Read the model definition and answer for the solid it produces. Units are mm, in the model's axes. Face numbers are marked on the shaded views. A direction names the side the tool comes from. Give positions to 0.01 mm unless a question says otherwise; leave off trailing zeros. Loops run counter-clockwise (first coordinate to the right, second up) from the corner with the lowest first, then second, coordinate; pieces in that order, holes last. Notation, with made-up numbers: (-10.5, -36.5) - (26.5, -36.5) arc R22 ccw to (26.5, 2.5) - close; hole circle Ø4 at (-7, 88.5). An arc over 180 degrees is marked (long way). Write each question's results on one line, items separated by ' | '. Start each with the question number.
Q1. The part is cut by section D-D, the plane z = -15. State how many separate pieces and enclosed holes the cut face has, plus the area to 3 significant figures.
Q2. The part is cut by section A-A, the plane y = 15.06. Write down the section's boundary in (x, z) (3 decimals).
Q3. The part is cut by section B-B, the plane x = 16.5. Write down the section's boundary in (y, z), plus the area to 3 significant figures.
Q4. For the marked faces 4, 5, 6, 7 and 8, determine the directions among +Z, -Z, +X, -X, +Y, -Y from which every point of the face is accessible in a straight line to the end or side of a thin tool.
Q5. Given pin 1 (1.5 mm diameter, centred on x = 31, z = -11.5, fed in from -Y); pin 2 (15 mm diameter, centred on y = 6.56, z = -15, fed in from -X); pin 3 (2 mm diameter, centred on y = 86, z = -27, fed in from -X); pin 4 (5.5 mm diameter, centred on y = 23.56, z = -15, fed in from -X), each flat-ended and moving along its own axis, determine where each tip first touches the part or whether it passes through.
Q6. Determine the mould class of the marked faces 1, 2 and 3 for opening direction Y: +Y half, -Y half, draft (parallel to the pull), parting line (faces both ways), or undercut.
Q7. The part is cut by section C-C, the plane z = 7.5. Write down the section's boundary in (x, y), plus the area to 3 significant figures.
Q8. Find the intervals of material crossed by line 1 (Y direction, x = 21, z = -15) (1 decimal); line 2 (Y direction, x = 26, z = -15) (3 decimals); line 3 (Z direction, x = 16, y = 18), in increasing order. Write a range as from..to.
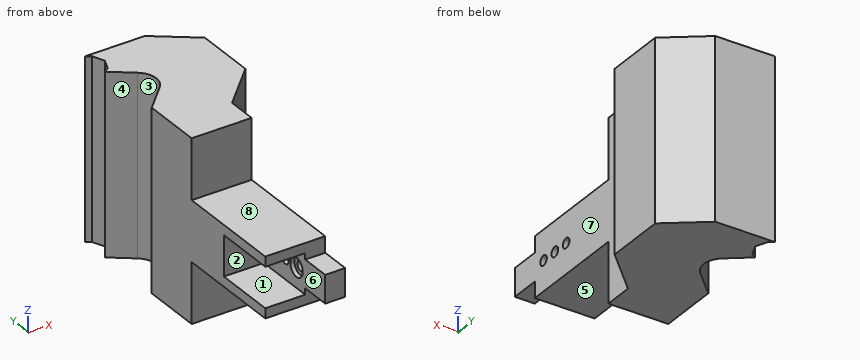
Autodesk Inventor part; units mm, degrees
ref_plane "Work Plane1" through (0, 0, -15) normal (0, 0, 1) x (1, 0, 0)
ref_plane "YZ Plane" through (0, 0, 0) normal (1, 0, 0) x (0, 1, 0)
ref_plane "XZ Plane" through (0, 0, 0) normal (0, 1, 0) x (-1, 0, 0)
sketch "Sketch1" plane through (0, 0, 0) normal (0, 0, 1) x (1, 0, 0)
  line L0 (0, 0) -> (25, 0)
  line L1 (25, 0) -> (25, 40)
  line L2 (25, 40) -> (0, 40)
  line L3 (0, 40) -> (0, 0)
  dimension "d1" = 25
  dimension "d2" = 40
  dimension "d3" = 25
extrude "Extrusion1" add sketch "Sketch1" against normal blind 30
sketch "Sketch2" plane through (25, 0, 0) normal (1, 0, 0) x (0, 0, -1)
  line L0 (0, 0) -> (30, 0)
  circle A0 centre (15, 6.56) radius 2.46
extrude "Extrusion2" cut sketch "Sketch2" against normal blind 30
sketch "Sketch3" plane through (0, 0, 0) normal (-1, 0, 0) x (0, 0, 1)
  line L0 (0, 0) -> (-30, 0)
  line L1 (-25.05, 0) -> (-4.95, 0)
  line L2 (-4.95, 0) -> (-4.95, 33.12)
  line L3 (-4.95, 33.12) -> (-25.05, 33.12)
  line L4 (-25.05, 33.12) -> (-25.05, 0)
  dimension "d11" = 20.1
extrude "Extrusion3" cut sketch "Sketch3" against normal blind 20
sketch "Sketch4" plane through (0, 0, 0) normal (0, -1, 0) x (1, 0, 0)
  line L0 (20, -4.95) -> (20, -25.05)
  line L1 (20, -15) -> (25, -15)
  line L2 (25, 0) -> (25, -30)
  line L3 (20, -8.025) -> (25, -8.025)
  line L4 (25, -8.025) -> (25, -21.975)
  line L5 (25, -21.975) -> (20, -21.975)
  line L6 (20, -21.975) -> (20, -8.025)
  line L7 (20, -8.025) -> (25, -21.975) construction
  line L8 (25, -8.025) -> (20, -21.975) construction
  line L9 (25, -12.54) -> (25, -17.46)
  point P0 (0, 0)
  point P1 (22.5, -15)
  dimension "d14" = 13.95
extrude "Extrusion4" add sketch "Sketch4" along normal blind 15
sketch "Sketch5" plane through (20, 0, 0) normal (-1, 0, 0) x (0, 0, 1)
  circle A0 centre (-15, 6.56) radius 2.46
  circle A1 centre (-15, 6.56) radius 4.7025
  circle A2 centre (-15, 6.56) radius 2.46
  circle A3 centre (-15, 6.56) radius 2.46
  point P0 (0, 0)
  dimension "d17" = 9.405
extrude "Extrusion5" cut sketch "Sketch5" against normal blind 2.1
sketch "Sketch6" plane through (25, 0, 0) normal (1, 0, 0) x (0, 0, -1)
  circle A0 centre (15, 6.56) radius 4.7025
  line L0 (15, 6.56) -> (15, 23.56)
  circle A1 centre (15, 23.56) radius 2.46
  point P0 (0, 0)
  dimension "d20" = 17
  dimension "d21" = 4.92
extrude "Extrusion6" cut sketch "Sketch6" against normal blind 10 contours A1
sketch "Sketch7" plane through (20, 0, 0) normal (-1, 0, 0) x (0, 0, 1)
  circle A0 centre (-15, 23.56) radius 2.46
  circle A1 centre (-15, 23.56) radius 4.7025
  point P0 (0, 0)
  dimension "d24" = 9.405
extrude "Extrusion7" cut sketch "Sketch7" against normal blind 2.1
sketch "Sketch9" plane through (25, 0, 0) normal (1, 0, 0) x (0, 0, -1)
  circle A0 centre (15, 6.56) radius 2.46
  circle A1 centre (15, 6.56) radius 2.46
  circle A2 centre (15, 23.56) radius 2.46
  circle A3 centre (15, 23.56) radius 2.46
  line L0 (30, 40) -> (30, 0)
  line L1 (30, 0) -> (30, 40)
  line L2 (30, 40) -> (0, 40)
  line L3 (0, 40) -> (0, 0)
  line L4 (0, 0) -> (8.025, 0)
  line L5 (21.975, 0) -> (21.975, -15)
  line L6 (21.975, -15) -> (8.025, -15)
  line L7 (8.025, -15) -> (8.025, 0)
  line L8 (0, 0) -> (8.025, 0)
  line L9 (21.975, 0) -> (30, 0)
extrude "Extrusion8" add sketch "Sketch9" along normal blind 5
sketch "Sketch10" plane through (0, 40, 0) normal (0, 1, 0) x (1, 0, 0)
  line L0 (0, 30) -> (30, 30)
  line L1 (30, 0) -> (0, 0)
  line L2 (0, 30) -> (30, 30)
  line L3 (30, 30) -> (30, 0)
  line L4 (30, 0) -> (0, 0)
  line L5 (0, 0) -> (0, 30)
extrude "Extrusion9" add sketch "Sketch10" along normal blind 30
sketch "Sketch12" plane through (30, 0, 0) normal (1, 0, 0) x (0, 0, -1)
  circle A0 centre (15, 6.56) radius 2.46
  line L0 (15, 6.56) -> (15, 15.06)
  circle A1 centre (15, 15.06) radius 2.525
  point P0 (0, 0)
  dimension "d31" = 8.5
  dimension "d33" = 5.05
extrude "Extrusion10" cut sketch "Sketch12" against normal blind 30 contours A1
sketch "Sketch15" plane through (0, 0, -25.05) normal (-1, 0, 0) x (0, 0, 1)
  line L0 (0, 33.12) -> (20.1, 33.12)
  line L1 (20.1, 33.12) -> (20.1, 0)
  line L2 (0, 33.12) -> (20.1, 33.12)
  line L3 (20.1, 33.12) -> (20.1, 31.1)
  line L4 (20.1, 31.1) -> (0, 31.1)
  line L5 (0, 31.1) -> (0, 33.12)
  point P0 (25.05, 0)
  dimension "d57" = 2.02
extrude "Extrusion13" add sketch "Sketch15" against normal blind 20
sketch "Sketch17" plane through (0, 0, 0) normal (0, 0, 1) x (1, 0, 0)
  line L0 (0, 70) -> (30, 70)
  line L1 (30, 70) -> (50.0622, 90.0622)
  line L2 (30, 70) -> (80, 70) construction
  line L3 (11.9522, 97.2454) -> (0, 85.2932)
  line L4 (0, 70) -> (0, 85.2932)
  line L5 (0, 70) -> (0, 0)
  line L6 (0, 70) -> (30, 70)
  line L7 (10.923, 112.2849) -> (0, 120.567)
  line L8 (2.5, 134.067) -> (0, 135.567)
  line L9 (2.5, 134.067) -> (5, 128.067)
  line L10 (2.5, 122.067) -> (0, 120.567)
  line L11 (2.5, 122.067) -> (5, 128.067)
  line L12 (50.0622, 105.3553) -> (50.0622, 120.567)
  line L13 (50.0622, 105.3553) -> (50.0622, 90.0622)
  line L14 (0, 135.567) -> (30, 135.567)
  line L15 (30, 135.567) -> (50.0622, 120.567)
  arc A0 (11.9522, 97.2454) -> (10.923, 112.2849) centre (4.8811, 104.3165) ccw
  dimension "d61" = 45
  dimension "d62" = 32.0271
  dimension "d71" = 30
  dimension "d72" = 10
extrude "Extrusion14" add sketch "Sketch17" against normal blind 30
sketch "Sketch19" plane through (0, 0, 0) normal (0, 0, 1) x (1, 0, 0)
  line L0 (30, 0) -> (30, 70)
  line L1 (30, 70) -> (50.0622, 90.0622)
  line L2 (30, 70) -> (50.0622, 90.0622)
  line L3 (50.0622, 120.567) -> (50.0622, 90.0622)
  line L4 (50.0622, 90.0622) -> (50.0622, 120.567)
  line L5 (30, 135.567) -> (50.0622, 120.567)
  line L6 (50.0622, 120.567) -> (30, 135.567)
  line L7 (0, 135.567) -> (30, 135.567)
  line L8 (30, 135.567) -> (0, 135.567)
  line L9 (5, 128.067) -> (2.5, 134.067)
  line L10 (0, 135.567) -> (2.5, 134.067)
  line L11 (2.5, 134.067) -> (5, 128.067)
  line L12 (2.5, 122.067) -> (5, 128.067)
  line L13 (5, 128.067) -> (2.5, 122.067)
  line L14 (0, 120.567) -> (2.5, 122.067)
  line L15 (2.5, 122.067) -> (0, 120.567)
  line L16 (10.923, 112.2849) -> (0, 120.567)
  line L17 (0, 120.567) -> (10.923, 112.2849)
  line L18 (11.9522, 97.2454) -> (0, 85.2932)
  line L19 (11.9522, 97.2454) -> (0, 85.2932)
  line L20 (0, 85.2932) -> (0, 55.2932)
  line L21 (0, 0) -> (0, 85.2932)
  line L22 (0, 55.2932) -> (30, 55.2932)
  line L23 (30, 55.2932) -> (30, 70)
  arc A0 (11.9522, 97.2454) -> (10.923, 112.2849) centre (4.8811, 104.3165) ccw
  dimension "d75" = 30
  dimension "d76" = 30
extrude "Extrusion15" add sketch "Sketch19" along normal blind 30
ref_plane "Work Plane1" through (0, 0, -15) normal (0, 0, 1) x (1, 0, 0)
mirror "Mirror1" about plane through (0, 0, -15) normal (0, 0, 1) of "Extrusion15"
properties part number "rec_c_12mm_x_90mm"
Check sheet entries:
1) separate pieces: 4 | enclosed holes: 0 | area: 4,020 mm^2
2) outline: (0, -30) - (30, -30) - (30, -17.525) - (20, -17.525) - (20, -25.05) - (0, -25.05) - close; (0, -4.95) - (20, -4.95) - (20, -12.475) - (30, -12.475) - (30, 0) - (0, 0) - close
3) outline: (0, -30) - (55.29, -30) - (55.29, -60) - (135.57, -60) - (135.57, 30) - (55.29, 30) - (55.29, 0) - (0, 0) - (0, -4.95) - (31.1, -4.95) - (31.1, -25.05) - (0, -25.05) - close | area: 8,260 mm^2
4) face 4: +Z, -Z, -X | face 5: -Z, +X, -X, -Y | face 6: -X, -Y | face 7: +Z, -Z, +X, -Y | face 8: +Z, +X, -X, -Y
5) pin 1: stops at y = 70.25 | pin 2: stops at x = 20 | pin 3: stops at x = 0 | pin 4: stops at x = 22.1
6) face 1: draft | face 2: -Y half | face 3: undercut
7) outline: (0, 55.29) - (30, 55.29) - (30, 70) - (50.06, 90.06) - (50.06, 120.57) - (30, 135.57) - (0, 135.57) - (2.5, 134.07) - (5, 128.07) - (2.5, 122.07) - (0, 120.57) - (10.92, 112.28) arc R10 cw to (11.95, 97.25) - (0, 85.29) - close | area: 3,000 mm^2
8) line 1: y = -15..1.9, 11.3..12.5, 17.6..18.9, 28.3..135.6 | line 2: y = -15..4.1, 9.02..12.535, 17.585..21.1, 26.02..135.567 | line 3: z = -30..-25.05, -4.95..0
